Geometry: see drawing. Coordinates: mm, zero at the bounding-box minimum. A direction names the side the tool comes from. Round coordinates to 2 decimals unless told otherwise and drop trailing zeros. Order: outer loops, then holes, each group sorted by start corner. A loop starts at its lowest first (then second) coordinate and runs counter-clockwise, first axis right, second up. Notation, with made-up numbers: (45.25, -4.5) -> (95.25, -4.5) arc R21 cw to (95.25, 32.5) -> close; hole circle Ø9 at (59, -25). An arc over 180 degrees is marked (long way). Put each result on its own line as item: value.
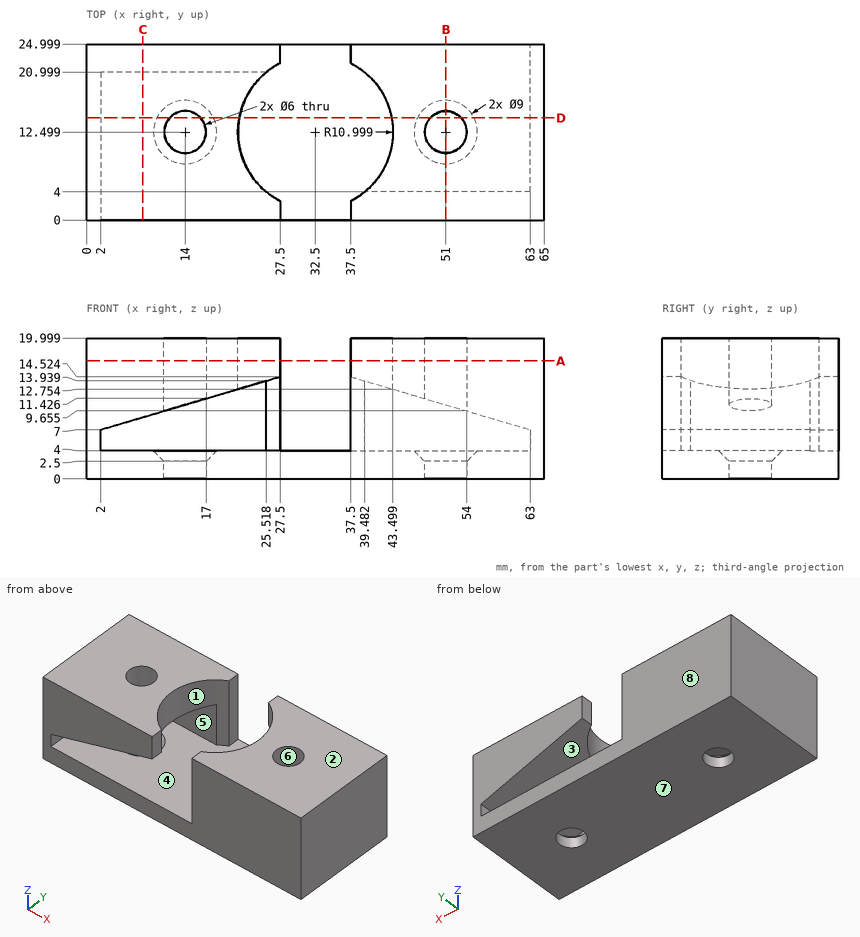
1. Cut plane C-C on x = 8. Return loops of the section in (y, z), and give its area (3 significant figures).
Ans:
outline: (0, 0) -> (25, 0) -> (25, 20) -> (0, 20) -> (0, 8.77) -> (21, 8.77) -> (21, 4) -> (0, 4) -> close
area: 400 mm²
2. Material intervals for probe 1 along Y at (x, z) = (51, 12.5); probe 2 along Y at (x, z) = (25, 8); probe 3 along Z at (x, y) = (34, 12.75), sorted ascending.
Ans:
probe 1: 0 to 9.5, 15.5 to 25
probe 2: 21 to 25
probe 3: 0 to 4
3. Contact query for flat-ended pins moving along their axis: P1, Ø3, axis at x = 19.5, z = 8.5, coming from the -Y side; P2, Ø3.5, axis at x = 51, y = 12.5, coming from the +Z side. Output: stop coordinate, or through.
Ans:
P1: y = 21
P2: through
4. Cut plane A-A on z = 16.75. Return loops of the section in (x, y), and give its area (3 significant figures).
Ans:
outline: (0, 0) -> (27.5, 0) -> (27.5, 2.7) arc R11 cw to (27.5, 22.3) -> (27.5, 25) -> (0, 25) -> close; (37.5, 0) -> (65, 0) -> (65, 25) -> (37.5, 25) -> (37.5, 22.3) arc R11 cw to (37.5, 2.7) -> close; hole circle Ø6 at (14, 12.5); hole circle Ø6 at (51, 12.5)
area: 1,150 mm²
5. Cut plane B-B on x = 51. Return loops of the section in (y, z).
Ans:
outline: (0, 0) -> (9.5, 0) -> (9.5, 2.5) -> (8, 4) -> (4, 4) -> (4, 10.54) -> (9.5, 10.54) -> (9.5, 20) -> (0, 20) -> close; (15.5, 0) -> (25, 0) -> (25, 4) -> (17, 4) -> (15.5, 2.5) -> close; (15.5, 10.54) -> (25, 10.54) -> (25, 20) -> (15.5, 20) -> close
6. Set-up query: the marked faces 1, 2, 3, 4 and 5. Return all of +Z, -Z, +X, -X, +Y, -Y with unobstructed straight access to the full face (end or side cutting, diameter ignored); none if empty.
Ans:
face 1: +Z
face 2: +Z, +X, -X, +Y, -Y
face 3: +Y
face 4: none
face 5: -Y
7. Cut plane D-D on y = 14.5. State how many separate pieces and enclosed holes the cut face has.
Ans:
separate pieces: 5
enclosed holes: 0
8. Draft query along Y for the marked faces 6, 7 and 8. Return one class per face: +Y half, -Y half, draft (parallel to the pull), parting line (faces both ways), or undercut.
Ans:
face 6: undercut
face 7: draft
face 8: +Y half
